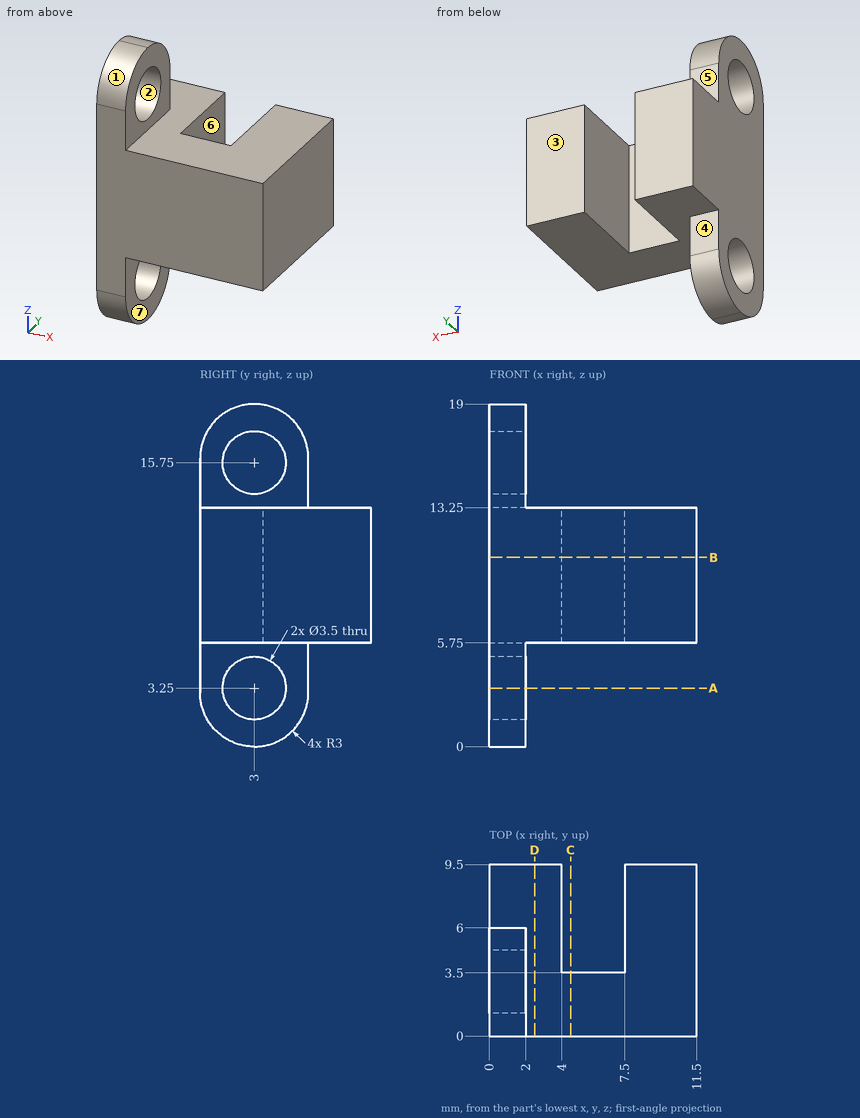
Input: dimensioned drawing with shaded views. Units: mm. Origin: part minimum x, y, z. A direction names the side the tool comes from. Coordinates: 2 decimals unless noted, no trailing zeros. Loops run counter-clockwise (first coordinate to the right, second up) from the corner with the lowest first, then second, coordinate; pieces in that order, holes last. Notation, with made-up numbers: M 55.5,16.25 L 114.5,16.25 A35 cw 114.5,55.25 Z; hole C 31,-4.75 d5. An arc over 180 degrees is marked long. One line per item, written item: value. Start each with the question number.
1) Cut plane D-D (x = 2.5). Return loops of the section in (y, z).
2) Reachability of the marked faces 4, 5, 6 and 7 from +Z, -Z, +X, -X, +Y, -Y: full face, straight path, thin tool, end or side. Return the list, or none.
3) Material intervals for L1, parallel to X at y = 5, z = 7.25; L2, parallel to Y at x = 1.55, z = 15.75; L3, parallel to Y at x = 5, z = 8.75, sorted ascending. Write a range as from..to.
4) Cut plane C-C (x = 4.5). Return loops of the section in (y, z), then the cut area to 4 significant figures.
5) Draft query along Z for the marked faces 1, 2 and 3. Return one class per face: released by +Z, released by -Z, zero draft, split by the parting line, or undercut.
6) Cut plane A-A (z = 3.25). Return loops of the section in (x, y).
7) Pin query (flat end, axial travel): P1, Ø5.5, axis at y = 3, z = 15.75, coming from the -X side; P2, Ø1, axis at x = 9.5, y = 7.5, coming from the -Z side; P3, Ø3, axis at x = 4, y = 3.5, coming from the +Z side; P4, Ø0.6, axis at x = 0.5, z = 14.5, coming from the +Y side. Return the tip coordinate at first contact, or that it passes through.
8) Cut plane B-B (z = 10.5). Return loops of the section in (x, y).
Evaluation:
1. outline: M 0,5.75 L 9.5,5.75 L 9.5,13.25 L 0,13.25 Z
2. face 4: -Z, +X, -X, +Y
2. face 5: +Z, +X, -X, +Y
2. face 6: +Z, -Z, +Y
2. face 7: -Z, +X, +Y, -Y
3. L1: 0..4, 7.5..11.5
3. L2: 0..1.25, 4.75..6
3. L3: 0..3.5
4. outline: M 0,5.75 L 3.5,5.75 L 3.5,13.25 L 0,13.25 Z
4. area: 26.25 mm^2
5. face 1: released by +Z
5. face 2: undercut
5. face 3: zero draft
6. outline: M 0,0 L 2,0 L 2,1.25 L 0,1.25 Z; M 0,4.75 L 2,4.75 L 2,6 L 0,6 Z
7. P1: x = 0
7. P2: z = 5.75
7. P3: z = 13.25
7. P4: y = 6
8. outline: M 0,0 L 11.5,0 L 11.5,9.5 L 7.5,9.5 L 7.5,3.5 L 4,3.5 L 4,9.5 L 0,9.5 Z
